from build123d import *

# Parameters (mm, degrees)
F0_R     = 2.75
F0_R_2   = 2
F1_DEPTH = 3
F2_DEPTH = 3


with BuildPart() as f1:
    # F0 (on Top) → F1 (new body)
    with BuildSketch(Plane.XY):
        with BuildLine():
            Line((-79.612069, -8.387931), (-79.612069, -22.387931))
            Line((-79.612069, -22.387931), (-79.612069, -37.387931))
            ThreePointArc((-79.612069, -37.387931), (-78.147603, -40.923465), (-74.612069, -42.387931))
            Line((-74.612069, -42.387931), (-64.612069, -42.387931))
            Line((-64.612069, -42.387931), (-52.612069, -42.387931))
            ThreePointArc((-52.612069, -42.387931), (-49.076535, -40.923465), (-47.612069, -37.387931))
            Line((-47.612069, -37.387931), (-47.612069, 36.612069))
            ThreePointArc((-47.612069, 36.612069), (-49.076535, 40.147603), (-52.612069, 41.612069))
            Line((-52.612069, 41.612069), (-64.612069, 41.612069))
            Line((-64.612069, 41.612069), (-67.112069, 41.612069))
            Line((-67.112069, 41.612069), (-74.612069, 41.612069))
            ThreePointArc((-74.612069, 41.612069), (-78.147603, 40.147603), (-79.612069, 36.612069))
            Line((-79.612069, 36.612069), (-79.612069, 21.612069))
            Line((-79.612069, 21.612069), (-79.612069, -8.387931))
        make_face()
        with Locations((-69.612069, -32.387931)):
            Circle(F0_R, mode=Mode.SUBTRACT)
        with Locations((-54.612069, -32.387931)):
            Circle(F0_R_2, mode=Mode.SUBTRACT)
        with Locations((-69.612069, 31.612069)):
            Circle(F0_R, mode=Mode.SUBTRACT)
        with Locations((-54.612069, 31.612069)):
            Circle(F0_R_2, mode=Mode.SUBTRACT)
    extrude(amount=F1_DEPTH)


with BuildPart() as f2:
    # F0 (on Top) → F2 (new body)
    with BuildSketch(Plane.XY):
        with BuildLine():
            Line((74.387931, -13.387931), (74.387931, -8.387931))
            Line((74.387931, -8.387931), (74.387931, 21.612069))
            Line((74.387931, 21.612069), (74.387931, 36.612069))
            ThreePointArc((74.387931, 36.612069), (72.923465, 40.147603), (69.387931, 41.612069))
            Line((69.387931, 41.612069), (59.387931, 41.612069))
            Line((59.387931, 41.612069), (52.387931, 41.612069))
            ThreePointArc((52.387931, 41.612069), (48.852397, 40.147603), (47.387931, 36.612069))
            Line((47.387931, 36.612069), (47.387931, -37.387931))
            ThreePointArc((47.387931, -37.387931), (48.852397, -40.923465), (52.387931, -42.387931))
            Line((52.387931, -42.387931), (59.387931, -42.387931))
            Line((59.387931, -42.387931), (69.387931, -42.387931))
            ThreePointArc((69.387931, -42.387931), (72.923465, -40.923465), (74.387931, -37.387931))
            Line((74.387931, -37.387931), (74.387931, -28.387931))
            Line((74.387931, -28.387931), (74.387931, -22.387931))
            Line((74.387931, -22.387931), (74.387931, -13.387931))
        make_face()
        with Locations((54.387931, -32.387931)):
            Circle(F0_R_2, mode=Mode.SUBTRACT)
        with Locations((64.387931, -32.387931)):
            Circle(F0_R, mode=Mode.SUBTRACT)
        with Locations((54.387931, 31.612069)):
            Circle(F0_R_2, mode=Mode.SUBTRACT)
        with Locations((64.387931, 31.612069)):
            Circle(F0_R, mode=Mode.SUBTRACT)
    extrude(amount=F2_DEPTH)


solid = f1.part
Could you check a few things on this model? Use its own coordinates, in mm. Give positions to 0.01 mm unless a question says otherwise; leave off trailing zeros. Order: outer loops, then holes, each group sorted by start corner. A loop starts at its lowest first (then second) coordinate and runs counter-clockwise, first axis right, second up. Notation, with made-up numbers: (-3, 36) -> (1, 36) arc R14 cw to (1, 45) -> close; hole circle Ø7 at (21.5, 57). An arc over 180 degrees is marked (long way). Return JSON: item names as keys, results as strings.
1. Imagine slicing it at A-A on x = -55.5. List the corners of the cut face in (y, z) for me, then the cut area to 3 significant figures.
Answer list:
{"outline": "(-42.39, 0) -> (-34.18, 0) -> (-34.18, 3) -> (-42.39, 3) -> close; (-30.6, 0) -> (29.82, 0) -> (29.82, 3) -> (-30.6, 3) -> close; (33.4, 0) -> (41.61, 0) -> (41.61, 3) -> (33.4, 3) -> close", "area": "230 mm2"}
2. Imagine slicing it at B-B on z = 0.8. List the corners of the cut face in (x, y) for me.
Answer list:
{"outline": "(-79.61, -37.39) arc R5 ccw to (-74.61, -42.39) -> (-52.61, -42.39) arc R5 ccw to (-47.61, -37.39) -> (-47.61, 36.61) arc R5 ccw to (-52.61, 41.61) -> (-74.61, 41.61) arc R5 ccw to (-79.61, 36.61) -> close; hole circle Ø5.5 at (-69.61, -32.39); hole circle Ø5.5 at (-69.61, 31.61); hole circle Ø4 at (-54.61, -32.39); hole circle Ø4 at (-54.61, 31.61)"}
3. I need wall thicknesses on line 1 (Y direction, x = -54.5, z = 0.85); line 2 (Y direction, x = -56, z = 1.25); line 3 (X direction, y = -33, z = 0.7). Which ranges of each line are inside material? Lowest first, please. Write a range as from..to.
Answer list:
{"line 1": "y = -42.39..-34.38, -30.39..29.62, 33.61..41.61", "line 2": "y = -42.39..-33.83, -30.95..30.17, 33.05..41.61", "line 3": "x = -79.61..-72.29, -66.93..-56.52, -52.71..-47.61"}
4. Imagine slicing it at C-C on x = -69.5. List the corners of the cut face in (y, z) for me, then the cut area to 3 significant figures.
Answer list:
{"outline": "(-42.39, 0) -> (-35.14, 0) -> (-35.14, 3) -> (-42.39, 3) -> close; (-29.64, 0) -> (28.86, 0) -> (28.86, 3) -> (-29.64, 3) -> close; (34.36, 0) -> (41.61, 0) -> (41.61, 3) -> (34.36, 3) -> close", "area": "219 mm2"}
5. Thinking about a two-plate mould opening in Y: for faces 1 (the flat face through (-63, 41.612, 1)), 2 (the flat face through (-64, 0, 0)), 3 (the flat face through (-64, -42.388, 1)), 4 (the cylindrical face through (-52.765, -33.154, 1.479)), which applies, pulls with the +Y half, pulls with the -Y half, needs draft (parallel to the pull), parting line crosses it, or undercut?
Answer list:
{"face 1": "pulls with the +Y half", "face 2": "needs draft", "face 3": "pulls with the -Y half", "face 4": "undercut"}
6. For pin 1 Ø3.5 at (x, y) = (-54.61, -32.39) entering from +Z, with a flat end and sliding along its axis, tell me the tip position at first contact or that it passes through.
Answer list:
{"pin 1": "passes through"}
